The model under review builds one solid part; all positions refer to its coordinate system, in mm. Face numbers are marked on the shaded views. Give positions to 0.01 mm unless a question says otherwise; leave off trailing zeros. Order: outer loops, then holes, each group sorted by start corner. A loop starts at its lowest first (then second) coordinate and runs counter-clockwise, first axis right, second up. Notation, with made-up numbers: (-29, 56.25) - (7, 56.25) arc R26 ccw to (7, 71.25) - close; hole circle Ø3 at (-2, 35). An arc over 180 degrees is marked (long way). Use a Markdown table: item, result. Add a question column.
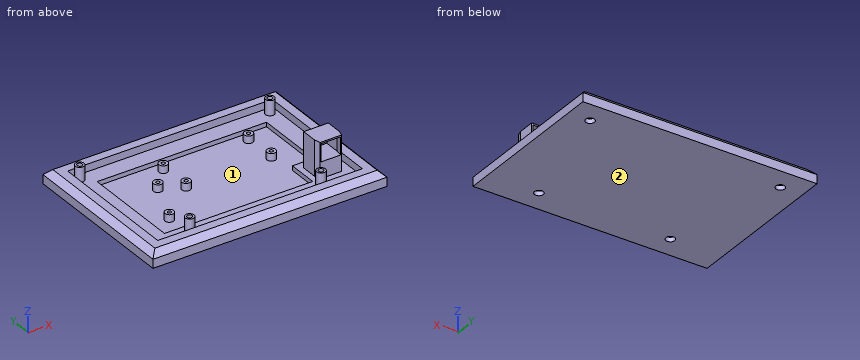
```python
from build123d import *

# Parameters (mm, degrees)
SKETCH_W        = 139.31
SKETCH_H        = 90.92
PAD_DEPTH       = 5
SKETCH001_R     = 1.75
POCKET_DEPTH    = 5.001
SKETCH002_R     = 3
POCKET001_DEPTH = 3
POCKET004_DEPTH = 3
SKETCH009_R     = 3
PAD003_DEPTH    = 5
SKETCH010_R     = 1.25
POCKET005_DEPTH = 5
PAD004_DEPTH    = 24
POCKET007_DEPTH = 6
SKETCH014_W     = 25
SKETCH014_H     = 11
POCKET008_DEPTH = 24.001
SKETCH015_W     = 159.31
SKETCH015_H     = 110.92
SKETCH015_W_2   = 139.31
SKETCH015_H_2   = 90.92
PAD005_DEPTH    = 10
SKETCH016_R     = 3
PAD006_DEPTH    = 10
SKETCH017_R     = 1.75
POCKET009_DEPTH = 15.001
CHAMFER_SIZE    = 4


with BuildPart() as part:
    # Sketch → Pad (new body)
    with BuildSketch(Plane.XY):
        Rectangle(SKETCH_W, SKETCH_H)
    extrude(amount=PAD_DEPTH)

    # Sketch001 (on Face5 of Pad) → Pocket (cut, through all)
    with BuildSketch(Plane(origin=(0, 0, 0), x_dir=(1, 0, 0), z_dir=(0, 0, -1))):
        with Locations((-44.735, 40.67)):
            Circle(SKETCH001_R)
        with Locations((-64.755, -40.56)):
            Circle(SKETCH001_R)
        with Locations((64.755, -40.56)):
            Circle(SKETCH001_R)
        with Locations((44.735, 40.67)):
            Circle(SKETCH001_R)
    extrude(amount=-POCKET_DEPTH, mode=Mode.SUBTRACT)

    # Sketch002 (on Face4 of Pocket) → Pocket001 (cut)
    with BuildSketch(Plane(origin=(0, 0, 0), x_dir=(1, 0, 0), z_dir=(0, 0, -1))):
        with Locations((-44.735, 40.67)):
            Circle(SKETCH002_R)
        with Locations((44.735, 40.67)):
            Circle(SKETCH002_R)
        with Locations((64.755, -40.56)):
            Circle(SKETCH002_R)
        with Locations((-64.755, -40.56)):
            Circle(SKETCH002_R)
    extrude(amount=-POCKET001_DEPTH, mode=Mode.SUBTRACT)

    # Sketch008 → Pocket004 (cut)
    with BuildSketch(Plane.XY.offset(5)):
        Polygon((-57.659628, -34.455423), (-57.659628, 33.450305), (57.659628, 33.450305), (57.659628, -13.955423), (43.279628, -13.955423), (43.279628, -34.455423), align=None)
    extrude(amount=-POCKET004_DEPTH, mode=Mode.SUBTRACT)

    # Sketch009 (on Face25 of Pocket004) → Pad003 (join)
    with BuildSketch(Plane.XY.offset(2)):
        with Locations((-44.159628, -19.455423)):
            Circle(SKETCH009_R)
        with Locations((-31.459628, 11.024577)):
            Circle(SKETCH009_R)
        with Locations((-17.340372, 26.450305)):
            Circle(SKETCH009_R)
        with Locations((-17.340372, 3.450305)):
            Circle(SKETCH009_R)
        with Locations((40.659628, 26.450305)):
            Circle(SKETCH009_R)
        with Locations((40.659628, 3.450305)):
            Circle(SKETCH009_R)
    extrude(amount=PAD003_DEPTH)

    # Sketch010 (on Face33 of Pad003) → Pocket005 (cut)
    with BuildSketch(Plane.XY.offset(7)):
        with Locations((-44.159628, -19.455423)):
            Circle(SKETCH010_R)
        with Locations((-31.459628, 11.024577)):
            Circle(SKETCH010_R)
        with Locations((-17.340372, 3.450305)):
            Circle(SKETCH010_R)
        with Locations((-17.340372, 26.450305)):
            Circle(SKETCH010_R)
        with Locations((40.659628, 26.450305)):
            Circle(SKETCH010_R)
        with Locations((40.659628, 3.450305)):
            Circle(SKETCH010_R)
    extrude(amount=-POCKET005_DEPTH, mode=Mode.SUBTRACT)

    # Sketch011 → Pad004 (join)
    with BuildSketch(Plane.XY.offset(5)):
        Polygon((61.655, -45.46), (49.655, -45.46), (49.655, -39.46), (47.28, -30.46), (47.28, -19.46), (64.03, -19.46), (64.03, -30.46), (61.655, -39.46), align=None)
    extrude(amount=PAD004_DEPTH)

    # Sketch013 → Pocket007 (cut, symmetric)
    with BuildSketch(Plane.XY.offset(22)):
        Polygon((48.355, -19.46), (62.955, -19.46), (62.955, -29.96), (60.655, -44.46), (50.655, -44.46), (48.355, -29.96), align=None)
    extrude(amount=POCKET007_DEPTH, both=True, mode=Mode.SUBTRACT)

    # Sketch014 (on Face5 of Pocket007) → Pocket008 (cut, through all)
    with BuildSketch(Plane.XY.offset(5)):
        with Locations((57.155, -39.96)):
            Rectangle(SKETCH014_W, SKETCH014_H)
    extrude(amount=POCKET008_DEPTH, mode=Mode.SUBTRACT)

    # Sketch015 → Pad005 (join)
    with BuildSketch(Plane.XY):
        Rectangle(SKETCH015_W, SKETCH015_H)
        Rectangle(SKETCH015_W_2, SKETCH015_H_2, mode=Mode.SUBTRACT)
    extrude(amount=PAD005_DEPTH)

    # Sketch016 (on Face10 of Pad005) → Pad006 (join)
    with BuildSketch(Plane.XY.offset(5)):
        with Locations((64.755, 40.56)):
            Circle(SKETCH016_R)
        with Locations((44.735, -40.67)):
            Circle(SKETCH016_R)
        with Locations((-44.735, -40.67)):
            Circle(SKETCH016_R)
        with Locations((-64.755, 40.56)):
            Circle(SKETCH016_R)
    extrude(amount=PAD006_DEPTH)

    # Sketch017 (on Face54 of Pad006) → Pocket009 (cut, through all)
    with BuildSketch(Plane.XY.offset(15)):
        with Locations((-64.755, 40.56)):
            Circle(SKETCH017_R)
        with Locations((64.755, 40.56)):
            Circle(SKETCH017_R)
        with Locations((44.735, -40.67)):
            Circle(SKETCH017_R)
        with Locations((-44.735, -40.67)):
            Circle(SKETCH017_R)
    extrude(amount=-POCKET009_DEPTH, mode=Mode.SUBTRACT)

    # Chamfer
    chamfer_edges = [part.edges().sort_by_distance(p)[0] for p in [
        (0, -55.46, 10),
        (-79.655, 0, 10),
        (0, 55.46, 10),
        (79.655, 0, 10),
    ]]
    chamfer(chamfer_edges, length=CHAMFER_SIZE)


solid = part.part
```
Q1. We need section D-D (y = 17.5). Write out the cut boundary in (x, z) (3 decimals).
Q2. We need section B-B (z = 19). Write out the cut boundary in (x, y) (3 decimals), plus the area to 3 significant figures.
Q3. Wall thickness on probe 1 along X at (y, z) = (-40.67, 1.3) (3 decimals); probe 2 along X at (y, z) = (40.56, 1.55) (3 decimals); probe 3 along X at (y, z) = (11, 5.25) (3 decimals): over which ranges is each line inside the solid? List them lowest first.
Q4. We need section C-C (x = 33). Write out the cut boundary in (y, z).
Q5. We need section A-A (y = -24.5). Write out the cut boundary in (x, z) (3 decimals), plus the area to 3 significant figures.
Q6. Clearance check with flat-ended pins moving along their axes: P1, Ø3, axis at x = 45.5, y = -39, coming from the -Z side; P2, Ø1.5, axis at x = 24, y = 9, coming from the +Z side; P3, Ø12, axis at y = -26, z = 15, coming from the +X side (3 decimals); P4, Ø9.5, axis at x = 64.755, y = 40.56, coming from the +Z side. State where each tip first meets the part, or that it passes through.
Q7. Draft analysis for pull direction Y (two halves, no side actions). For the marked faces 1 and 2, state which applies: pulls with the +Y half, pulls with the -Y half, needs draft (parallel to the pull), parting line crosses it, or undercut.
Here are the results:
| question | item | result |
|---|---|---|
| 1 | outline | (-79.655, 0) - (79.655, 0) - (79.655, 6) - (75.655, 10) - (69.655, 10) - (69.655, 5) - (57.66, 5) - (57.66, 2) - (-57.66, 2) - (-57.66, 5) - (-69.655, 5) - (-69.655, 10) - (-75.655, 10) - (-79.655, 6) - close |
| 2 | outline | (47.28, -30.46) - (48.336, -34.46) - (49.069, -34.46) - (48.355, -29.96) - (48.355, -19.46) - (47.28, -19.46) - close; (62.241, -34.46) - (62.974, -34.46) - (64.03, -30.46) - (64.03, -19.46) - (62.955, -19.46) - (62.955, -29.96) - close |
| 2 | area | 31.2 mm2 |
| 3 | probe 1 | -79.655 to -47.735, -41.735 to 41.735, 47.735 to 79.655 |
| 3 | probe 2 | -79.655 to -67.755, -61.755 to 61.755, 67.755 to 79.655 |
| 3 | probe 3 | -79.655 to -69.655, -34.46 to -32.709, -30.21 to -28.46, 69.655 to 79.655 |
| 4 | outline | (-55.46, 0) - (55.46, 0) - (55.46, 6) - (51.46, 10) - (45.46, 10) - (45.46, 5) - (33.45, 5) - (33.45, 2) - (-34.46, 2) - (-34.46, 5) - (-45.46, 5) - (-45.46, 10) - (-51.46, 10) - (-55.46, 6) - close |
| 5 | outline | (-79.655, 0) - (79.655, 0) - (79.655, 6) - (75.655, 10) - (69.655, 10) - (69.655, 5) - (64.03, 5) - (64.03, 29) - (47.28, 29) - (47.28, 5) - (43.28, 5) - (43.28, 2) - (-57.66, 2) - (-57.66, 5) - (-69.655, 5) - (-69.655, 10) - (-75.655, 10) - (-79.655, 6) - close; hole (48.355, 16) - (62.955, 16) - (62.955, 28) - (48.355, 28) - close |
| 5 | area | 805 mm2 |
| 6 | P1 | z = 0 |
| 6 | P2 | z = 2 |
| 6 | P3 | x = 76.655 |
| 6 | P4 | z = 15 |
| 7 | face 1 | undercut |
| 7 | face 2 | needs draft |
